```python
from build123d import *

# Parameters (mm, degrees)
F0_R     = 38.1
F1_DEPTH = 12.7
F2_R     = 3.175
F3_DEPTH = 6.35
F4_R     = 25.4
F5_DEPTH = 12.7
F6_R     = 12.7
F7_DEPTH = 25.4
F7_TAPER = 5
F8_R     = 5.08
F9_R     = 10.16


with BuildPart() as f1:
    # F0 (on Top) → F1 (new body)
    with BuildSketch(Plane.XY):
        with Locations((0.9899509557, 0)):
            Circle(F0_R)
    extrude(amount=F1_DEPTH)

    # F2 (on face) → F3 (cut)
    with BuildSketch(Plane(origin=(0, 0, 0), x_dir=(1, 0, 0), z_dir=(0, 0, -1))):
        with Locations((-19.05, -19.05)):
            Circle(F2_R)
        with Locations((19.05, -19.05)):
            Circle(F2_R)
        with Locations((19.05, 19.05)):
            Circle(F2_R)
        with Locations((-19.05, 19.05)):
            Circle(F2_R)
    extrude(amount=-F3_DEPTH, mode=Mode.SUBTRACT)

    # F4 (on face) → F5 (join)
    with BuildSketch(Plane.XY.offset(12.7)):
        Circle(F4_R)
    extrude(amount=F5_DEPTH)

    # F6 (on face) → F7 (join)
    with BuildSketch(Plane.XY.offset(25.4)):
        Circle(F6_R)
    extrude(amount=F7_DEPTH, taper=F7_TAPER)

    # F8
    f8_edges = [f1.edges().sort_by_distance(p)[0] for p in [
        (-37.110049, 0, 12.7),
        (-25.4, 0, 12.7),
        (-25.4, 0, 25.4),
        (-12.7, 0, 25.4),
    ]]
    fillet(f8_edges, radius=F8_R)

    # F9
    f9_edges = [f1.edges().sort_by_distance(p)[0] for p in [
        (-10.477788, 0, 50.8),
    ]]
    fillet(f9_edges, radius=F9_R)


solid = f1.part
```
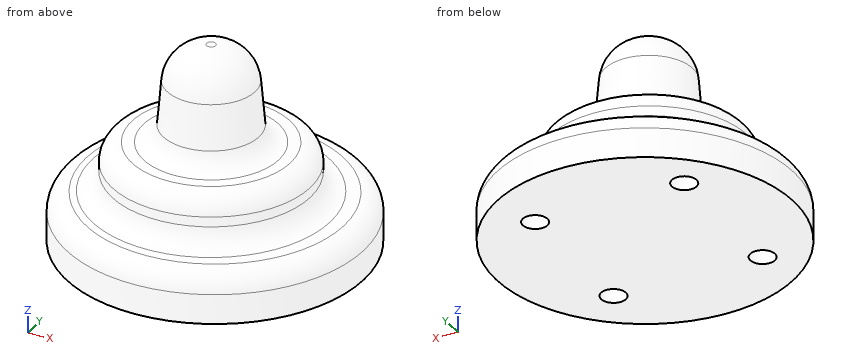
Part model, mm, in its own coordinate system. Round coordinates to 2 decimals unless told otherwise and drop trailing zeros. Order: outer loops, then holes, each group sorted by start corner. A loop starts at its lowest first (then second) coordinate and runs counter-clockwise, first axis right, second up. Notation, with made-up numbers: M 85.25,78.25 L 128.25,78.25 A23 ccw 128.25,108.25 Z; hole C 43,29.5 d3. An arc over 180 degrees is marked long. Put each result on its own line as item: value. Start each with the question number.
1. Slice it at B-B on z = 16. List the corners of the cut face in (x, y).
2. Drill centre lines: probe 1 along X at (y, z) = (19, 2); probe 2 along Y at (x, z) = (19, 2); probe 3 along Y at (x, z) = (-19.05, 3) (3 decimals). Where is each one in solid material? Low to high. Write a range as [from, to].
3. Drop flat-ended pins along their axis: pin 1 (8 mm diameter, centred on x = -8, z = 27.5, fed in from -Y); pin 2 (5.5 mm diameter, centred on x = 19.05, y = -19.05, fed in from -Z); pin 3 (10 mm diameter, centred on x = 9, y = 0.5, fed in from -Z); pin 4 (10 mm diameter, centred on y = 28.5, z = 18, fed in from +X). Give the stop position or say it passes through.
4. Slice it at A-A on z = 9. List the corners of the cut face in (x, y).
Findings:
1. outline: C 0,0 d51.44
2. probe 1: [-32.03, -22.22], [-15.88, 15.88], [22.22, 34.01]
2. probe 2: [-33.57, -22.22], [-15.88, 15.88], [22.22, 33.57]
2. probe 3: [-32.404, -22.225], [-15.875, 15.875], [22.225, 32.404]
3. pin 1: y = -23.15
3. pin 2: z = 6.35
3. pin 3: z = 0
3. pin 4: x = 9.64
4. outline: C 0.99,0 d75.82
